For this review, use the dimensioned drawing (mm, ordinates from the lowest corner) and the shaded views. A direction names the side the tool comes from. Round coordinates to 2 decimals unless told otherwise and drop trailing zeros. Loops run counter-clockwise (first coordinate to the right, second up) from the corner with the lowest first, then second, coordinate; pieces in that order, holes last. Notation, with made-up numbers: (68, -11) - (90, -11) arc R20 ccw to (90, -4) - close; hole circle Ø9 at (-10.75, 61). An arc over 180 degrees is marked (long way). Use one line per item in the form item = value. Start each with the question number.
(1) Wall thickness on probe 1 along X at (y, z) = (2.2, 4); probe 2 along X at (y, z) = (0.95, 5); probe 3 along X at (y, z) = (1.65, 13): over which ranges is each line inside the solid? List them lowest first. Write a range as [from, to].
(2) We need section D-D, the plane z = 10.25. Write out the cut boundary in (x, y).
(3) We need section A-A, the plane x = 9. Write out the cut boundary in (y, z), then the cut area to 3 significant figures.
(4) The part is to be moulded in two halves that separate along Z. For the marked faces 1, 2, 3 and 4, say which applies: released by +Z, released by -Z, zero draft, split by the parting line, or undercut.
(5) We need section C-C, the plane y = 1.95. Write out the cut boundary in (x, z).
(6) We need section B-B, the plane z = 4. Write out the cut boundary in (x, y), then the cut area to 3 significant figures.
(7) For pin 1 (2 mm diameter, centred on y = 1, z = 12.5, fed in from +X), flat-tipped, find the tip position at first contact; note if it passes through.
(8) Machinability: for the marked faces 5, 6 and 7, which of the approach directions +Z, -Z, +X, -X, +Y, -Y give a long, thin tool a straight path to every point of the face, cutting with its end or side? Answer none if there is none.
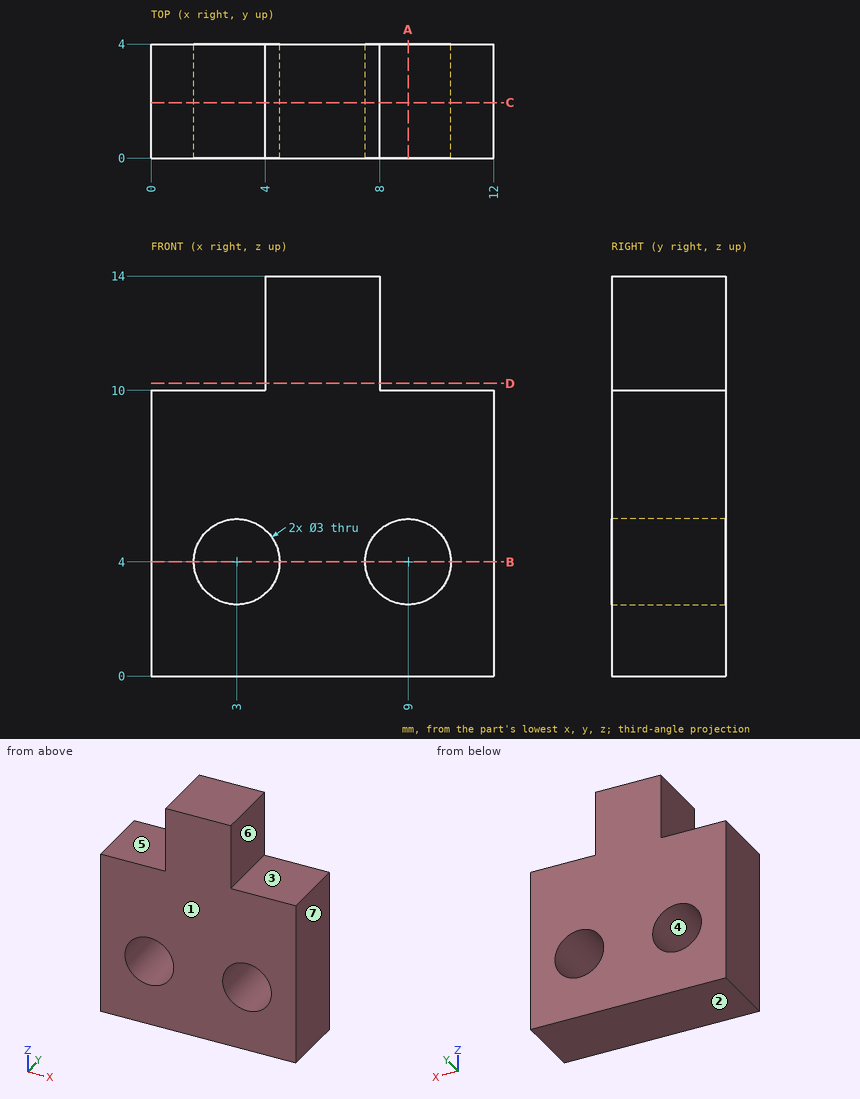
Data:
q1.probe_1 = [0, 1.5], [4.5, 7.5], [10.5, 12]
q1.probe_2 = [0, 1.88], [4.12, 7.88], [10.12, 12]
q1.probe_3 = [4, 8]
q2.outline = (4, 0) - (8, 0) - (8, 4) - (4, 4) - close
q3.outline = (0, 0) - (4, 0) - (4, 2.5) - (0, 2.5) - close; (0, 5.5) - (4, 5.5) - (4, 10) - (0, 10) - close
q3.area = 28.0 mm^2
q4.face_1 = zero draft
q4.face_2 = released by -Z
q4.face_3 = released by +Z
q4.face_4 = undercut
q5.outline = (0, 0) - (12, 0) - (12, 10) - (8, 10) - (8, 14) - (4, 14) - (4, 10) - (0, 10) - close; hole circle Ø3 at (3, 4); hole circle Ø3 at (9, 4)
q6.outline = (0, 0) - (1.5, 0) - (1.5, 4) - (0, 4) - close; (4.5, 0) - (7.5, 0) - (7.5, 4) - (4.5, 4) - close; (10.5, 0) - (12, 0) - (12, 4) - (10.5, 4) - close
q6.area = 24.0 mm^2
q7.pin_1 = 8
q8.face_5 = +Z, -X, +Y, -Y
q8.face_6 = +Z, +X, +Y, -Y
q8.face_7 = +Z, -Z, +X, +Y, -Y
